Autodesk Inventor part; units mm, degrees
ref_plane "YZ Plane" through (0, 0, 0) normal (1, 0, 0) x (0, 1, 0)
ref_plane "XZ Plane" through (0, 0, 0) normal (0, 1, 0) x (-1, 0, 0)
ref_plane "XY Plane" through (0, 0, 0) normal (0, 0, 1) x (1, 0, 0)
sketch "Sketch1" plane through (0, 0, 0) normal (0, 0, 1) x (1, 0, 0)
  line L0 (38.1, -38.1) -> (-38.1, -38.1)
  line L1 (-38.1, -38.1) -> (-38.1, 38.1)
  line L2 (-38.1, 38.1) -> (38.1, 38.1)
  line L3 (38.1, 38.1) -> (38.1, -38.1)
  line L4 (38.1, -38.1) -> (-38.1, 38.1) construction
  line L5 (-38.1, -38.1) -> (38.1, 38.1) construction
  line L6 (-34.925, -34.925) -> (34.925, -34.925)
  line L7 (34.925, -34.925) -> (34.925, 34.925)
  line L8 (34.925, 34.925) -> (-34.925, 34.925)
  line L9 (-34.925, 34.925) -> (-34.925, -34.925)
  line L10 (-34.925, -34.925) -> (34.925, 34.925) construction
  line L11 (34.925, -34.925) -> (-34.925, 34.925) construction
  point P0 (0, 0)
  dimension "d0" = 76.2
  dimension "d1" = 76.2
  dimension "d2" = 69.85
  dimension "d3" = 69.85
extrude "Extrusion1" add sketch "Sketch1" along normal blind 6.35 contours L0 L1 L2 L3 | L9 L8 L7 L6
extrude "Extrusion2" add sketch "Sketch1" along normal blind 38.1
fillet "Fillet1" radius 3.175 8 edges at (0, 38.1, 0) (38.1, 0, 0) (-38.1, 0, 0) (0, -38.1, 0) (38.1, 38.1, 19.05) (-38.1, 38.1, 19.05) (38.1, -38.1, 19.05) (-38.1, -38.1, 19.05)
sketch "Sketch2" plane through (0, 0, 6.35) normal (0, 0, 1) x (1, 0, 0)
  circle A0 centre (0, 0) radius 20.32
  circle A1 centre (0, 0) radius 21.9075
  dimension "d9" = 40.64
  dimension "d10" = 43.815
extrude "Extrusion3" add sketch "Sketch2" along normal blind 19.05
sketch "Sketch3" plane through (0, 0, 6.35) normal (0, 0, 1) x (1, 0, 0)
  line L0 (-25.4, -25.4) -> (25.4, -25.4)
  line L1 (25.4, -25.4) -> (25.4, 25.4)
  line L2 (25.4, 25.4) -> (-25.4, 25.4)
  line L3 (-25.4, 25.4) -> (-25.4, -25.4)
  line L4 (-25.4, -25.4) -> (25.4, 25.4) construction
  line L5 (25.4, -25.4) -> (-25.4, 25.4) construction
  circle A0 centre (25.4, 25.4) radius 3.175
  circle A1 centre (-25.4, 25.4) radius 3.175
  circle A2 centre (-25.4, -25.4) radius 3.175
  circle A3 centre (25.4, -25.4) radius 3.175
  point P0 (0, 0)
  dimension "d13" = 50.8
  dimension "d14" = 50.8
  dimension "d15" = 6.35
  dimension "d16" = 6.35
  dimension "d17" = 6.35
  dimension "d18" = 6.35
extrude "Extrusion4" add sketch "Sketch3" along normal blind 76.2 contours L3 A2 L0 | L0 A2 L3 | A3 L1 L0 | L0 L1 A3 | A1 L2 L3 | L3 L2 A1 | A0 L2 L1 | L1 L2 A0
sketch "Sketch4" plane through (25.4, 25.4, 82.55) normal (0, 0, 1) x (1, 0, 0)
  line L0 (0, 0) -> (-3.175, 0)
  circle A0 centre (-50.8, -50.8) radius 3.175
  circle A1 centre (0, -50.8) radius 3.175
  circle A2 centre (0, 0) radius 3.175
  circle A3 centre (-50.8, 0) radius 3.175
  circle A4 centre (-50.8, -50.8) radius 3.175
  line L1 (-50.8, -47.625) -> (-47.625, -50.8)
  line L2 (1.5875, -1.5875) -> (-1.5875, 1.5875)
  circle A5 centre (-50.8, 0) radius 3.175
  line L3 (-1.5875, -52.3875) -> (1.5875, -49.2125)
  line L4 (-38.862, -42.037) -> (-11.938, -42.037)
  line L5 (-8.763, -38.862) -> (-8.763, -11.938)
  line L6 (-11.938, -8.763) -> (-38.862, -8.763)
  line L7 (-42.037, -11.938) -> (-42.037, -38.862)
  line L8 (-42.037, -42.037) -> (-8.763, -8.763) construction
  line L9 (-8.763, -42.037) -> (-42.037, -8.763) construction
  line L10 (-11.0316, -39.7684) -> (-39.7684, -39.7684)
  line L11 (-39.7684, -39.7684) -> (-39.7684, -11.0316)
  line L12 (-39.7684, -11.0316) -> (-11.0316, -11.0316)
  line L13 (-11.0316, -11.0316) -> (-11.0316, -39.7684)
  line L14 (-11.0316, -39.7684) -> (-39.7684, -11.0316) construction
  line L15 (-39.7684, -39.7684) -> (-11.0316, -11.0316) construction
  line L16 (-50.8, -3.175) -> (-42.037, -11.938)
  line L17 (1.5875, -49.2125) -> (-8.763, -38.862)
  line L18 (-38.862, -8.763) -> (-47.625, 0)
  line L19 (-8.763, -11.938) -> (1.5875, -1.5875)
  line L20 (-1.5875, 1.5875) -> (-11.938, -8.763)
  line L21 (-42.037, -38.862) -> (-50.8, -47.625)
  line L22 (-47.625, -50.8) -> (-38.862, -42.037)
  line L23 (-11.938, -42.037) -> (-1.5875, -52.3875)
  line L24 (0, -50.8) -> (0, -47.625)
  line L25 (0, -3.175) -> (0, 0)
  line L26 (-50.8, -50.8) -> (-47.625, -50.8)
  line L27 (-3.175, -50.8) -> (0, -50.8)
  line L28 (-50.8, 0) -> (-50.8, -3.175)
  line L29 (-50.8, -47.625) -> (-50.8, -50.8)
  line L30 (-8.763, -11.938) -> (-8.763, -8.763)
  line L31 (-11.938, -8.763) -> (-8.763, -8.763)
  line L32 (-38.862, -8.763) -> (-42.037, -8.763)
  line L33 (-42.037, -11.938) -> (-42.037, -8.763)
  line L34 (-42.037, -38.862) -> (-42.037, -42.037)
  line L35 (-38.862, -42.037) -> (-42.037, -42.037)
  line L36 (-11.938, -42.037) -> (-8.763, -42.037)
  line L37 (-8.763, -42.037) -> (-8.763, -38.862)
  point P0 (-25.4, -25.4)
  point P1 (-25.4, -25.4)
  point P2 (-47.625, 0)
  point P3 (-3.175, -50.8)
  point P4 (0, -47.625)
  point P5 (0, -3.175)
  point P6 (-3.175, 0)
  dimension "d21" = 50.8
  dimension "d22" = 50.8
  dimension "d23" = 33.274
  dimension "d24" = 33.274
extrude "Extrusion5" add sketch "Sketch4" along normal blind 6.35
extrude "Extrusion6" add sketch "Sketch4" along normal blind 12.7 contours L31 L30 L5 L37 L36 L4 L35 L34 L7 L33 L32 L6
sketch "Sketch5" plane through (25.4, 25.4, 95.25) normal (0, 0, 1) x (1, 0, 0)
  circle A0 centre (-25.4, -25.4) radius 20.32
  line L0 (-39.7495, -11.0127) -> (-11.0505, -11.0127)
  line L1 (-11.0505, -11.0127) -> (-11.0505, -39.7873)
  line L2 (-11.0505, -39.7873) -> (-39.7495, -39.7873)
  line L3 (-39.7495, -39.7873) -> (-39.7495, -11.0127)
  line L4 (-39.7495, -11.0127) -> (-11.0505, -39.7873) construction
  line L5 (-11.0505, -11.0127) -> (-39.7495, -39.7873) construction
  line L6 (-34.925, -34.925) -> (-15.875, -34.925)
  line L7 (-15.875, -34.925) -> (-15.875, -15.875)
  line L8 (-15.875, -15.875) -> (-34.925, -15.875)
  line L9 (-34.925, -15.875) -> (-34.925, -34.925)
  line L10 (-34.925, -34.925) -> (-15.875, -15.875) construction
  line L11 (-15.875, -34.925) -> (-34.925, -15.875) construction
  line L12 (-14.2875, -36.5125) -> (-36.5125, -36.5125)
  line L13 (-36.5125, -36.5125) -> (-36.5125, -14.2875)
  line L14 (-36.5125, -14.2875) -> (-14.2875, -14.2875)
  line L15 (-14.2875, -14.2875) -> (-14.2875, -36.5125)
  line L16 (-14.2875, -36.5125) -> (-36.5125, -14.2875) construction
  line L17 (-36.5125, -36.5125) -> (-14.2875, -14.2875) construction
  dimension "d29" = 19.05
  dimension "d30" = 19.05
  dimension "d33" = 22.225
  dimension "d34" = 22.225
extrude "Extrusion8" add sketch "Sketch5" against normal blind 6.35 contours L1 L2 L3 L0 | L12 L13 L14 L15
extrude "Extrusion9" add sketch "Sketch5" along normal blind 6.35 contours L12 L13 L14 L15
sketch "Sketch6" plane through (25.4, 25.4, 101.6) normal (0, 0, 1) x (1, 0, 0)
  line L0 (-14.2875, -36.5125) -> (-36.5125, -36.5125)
  line L1 (-36.5125, -14.2875) -> (-14.2875, -14.2875)
  line L2 (-14.2875, -14.2875) -> (-14.2875, -36.5125)
  line L3 (-14.2875, -36.5125) -> (-36.5125, -36.5125)
  line L4 (-36.5125, -36.5125) -> (-36.5125, -14.2875)
  line L5 (-36.5125, -14.2875) -> (-14.2875, -36.5125) construction
  line L6 (-14.2875, -14.2875) -> (-36.5125, -36.5125) construction
  line L7 (-39.6875, -11.1125) -> (-11.1125, -11.1125)
  line L8 (-11.1125, -11.1125) -> (-11.1125, -39.6875)
  line L9 (-11.1125, -39.6875) -> (-39.6875, -39.6875)
  line L10 (-39.6875, -39.6875) -> (-39.6875, -11.1125)
  line L11 (-39.6875, -11.1125) -> (-11.1125, -39.6875) construction
  line L12 (-11.1125, -11.1125) -> (-39.6875, -39.6875) construction
  point P0 (-25.4, -25.4)
  dimension "d39" = 28.575
  dimension "d40" = 28.575
extrude "Extrusion10" add sketch "Sketch6" against normal blind 3.175
equation "\"d34\" = d33"
properties part number "Hot Air Ballon"
For this review, take the finished solid that the model builds, in its own axes (mm). A direction names the side the tool comes from. Give positions to 0.01 mm unless a question says otherwise; leave off trailing zeros. Loops run counter-clockwise (first coordinate to the right, second up) from the corner with the lowest first, then second, coordinate; pieces in that order, holes last.
Item 1: Insertion check: pin 1 (2.5 mm diameter, centred on x = 2.5, z = 100, fed in from +Y); pin 2 (6.5 mm diameter, centred on y = 5.5, z = 87, fed in from -X); pin 3 (4 mm diameter, centred on x = 2.5, z = 92.5, fed in from +Y). Each pin has a flat end and moves straight along its axis. Give the tip position at first contact, or say it passes through.
Item 2: For line 1 along Y through (x, z) = (0, 12.75) (1 decimal); line 2 along Z through (x, y) = (11, 12.5) (3 decimals); line 3 along Z through (x, y) = (20, 21.5), list the stretches that pass through material, from the lowest coordinate up.
Item 3: Take a section at D-D, the plane z = 73. State the section outline as (x, y) points (3 decimals).
Item 4: Tool access review of faces 1 (the flat face through (0, -11.112, 97)), 2 (the flat face through (-16.637, 0, 89)), 3 (the flat face through (0, 14.368, 86)): name each direction out of +Z, -Z, +X, -X, +Y, -Y from which nothing blocks a thin tool from reaching the whole face with its end or side.
Item 5: Take a section at C-C, the plane z = 86.5. State the section outline as (x, y) points (3 decimals).
Item 6: Take a section at A-A, the plane z = 9. Give the number of separate pieces and of enclosed holes in the cut face, and give its area (3 significant figures).
Item 7: Draft analysis for pull direction X (two halves, no side actions). For faces 4 (the flat face through (17.905, 21.08, 85.681)), 5 (the flat face through (-20.957, -17.782, 85.681)), 6 (the flat face through (11.112, 0, 97)), state which applies: +X half, -X half, draft (parallel to the pull), parting line (faces both ways), or undercut.
Item 8: Take a section at B-B, the plane z = 27.5. State the section outline as (x, y) points (3 decimals), and give its area (3 significant figures).
Calculated:
1. pin 1: stops at y = 14.29
1. pin 2: stops at x = -16.64
1. pin 3: stops at y = 16.64
2. line 1: y = -38.1 to -34.9, -21.9 to -20.3, 20.3 to 21.9, 34.9 to 38.1
2. line 2: z = 0 to 6.35, 88.9 to 95.25, 98.425 to 101.6
2. line 3: z = 0 to 6.35, 82.55 to 88.9
3. outline: circle Ø6.35 at (-25.4, -25.4); circle Ø6.35 at (-25.4, 25.4); circle Ø6.35 at (25.4, -25.4); circle Ø6.35 at (25.4, 25.4)
4. face 1: +X, -X, -Y
4. face 2: +Z, -X
4. face 3: none
5. outline: (-25.4, -22.225) arc R3.175 ccw (long way) to (-22.225, -25.4) - (-13.462, -16.637) - (13.462, -16.637) - (22.225, -25.4) arc R3.175 ccw (long way) to (25.4, -22.225) - (16.637, -13.462) - (16.637, 13.462) - (25.4, 22.225) arc R3.175 ccw (long way) to (22.225, 25.4) - (13.462, 16.637) - (-13.462, 16.637) - (-22.225, 25.4) arc R3.175 ccw (long way) to (-25.4, 22.225) - (-16.637, 13.462) - (-16.637, -13.462) - close; hole (-14.368, -14.368) - (14.368, -14.368) - (14.368, 14.368) - (-14.368, 14.368) - close
6. separate pieces: 6
6. enclosed holes: 2
6. area: 1,260 mm2
7. face 4: undercut
7. face 5: -X half
7. face 6: +X half
8. outline: (-38.1, -34.925) arc R3.175 ccw to (-34.925, -38.1) - (34.925, -38.1) arc R3.175 ccw to (38.1, -34.925) - (38.1, 34.925) arc R3.175 ccw to (34.925, 38.1) - (-34.925, 38.1) arc R3.175 ccw to (-38.1, 34.925) - close; circle Ø6.35 at (-25.4, -25.4); circle Ø6.35 at (-25.4, 25.4); circle Ø6.35 at (25.4, -25.4); circle Ø6.35 at (25.4, 25.4); hole (-34.925, -34.925) - (34.925, -34.925) - (34.925, 34.925) - (-34.925, 34.925) - close
8. area: 1,050 mm2
